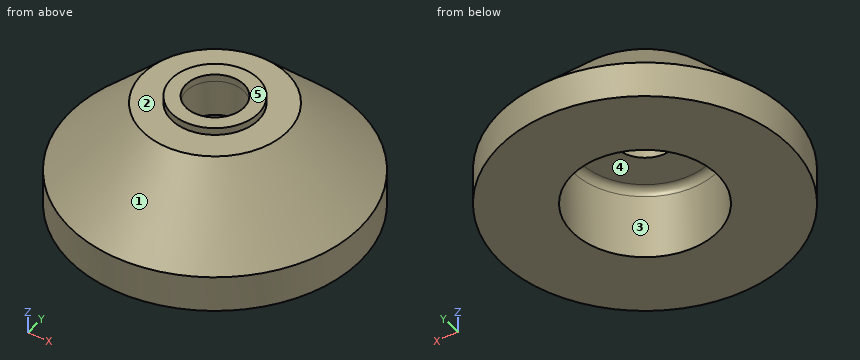
from build123d import *

# Parameters (mm, degrees)
F0_R     = 20
F1_DEPTH = 15
F2_SIZE  = 10
F3_R     = 6
F3_R_2   = 4
F4_DEPTH = 1
F5_R     = 4
F6_DEPTH = 15.001
F7_R     = 10
F8_DEPTH = 10
F9_R     = 1


with BuildPart() as f1:
    # F0 (on Top) → F1 (new body)
    with BuildSketch(Plane.XY):
        Circle(F0_R)
    extrude(amount=F1_DEPTH)

    # F2
    f2_edges = [f1.edges().sort_by_distance(p)[0] for p in [
        (-20, 0, 15),
    ]]
    chamfer(f2_edges, length=F2_SIZE)

    # F3 (on face) → F4 (join)
    with BuildSketch(Plane.XY.offset(15)):
        Circle(F3_R)
        Circle(F3_R_2, mode=Mode.SUBTRACT)
    extrude(amount=F4_DEPTH)

    # F5 (on face) → F6 (cut, through all)
    with BuildSketch(Plane.XY.offset(15)):
        Circle(F5_R)
    extrude(amount=-F6_DEPTH, mode=Mode.SUBTRACT)

    # F7 (on face) → F8 (cut)
    with BuildSketch(Plane(origin=(0, 0, 0), x_dir=(1, 0, 0), z_dir=(0, 0, -1))):
        Circle(F7_R)
    extrude(amount=-F8_DEPTH, mode=Mode.SUBTRACT)

    # F9
    f9_edges = [f1.edges().sort_by_distance(p)[0] for p in [
        (-10, 0, 10),
    ]]
    fillet(f9_edges, radius=F9_R)


solid = f1.part
The model under review builds one solid part; all positions refer to its coordinate system, in mm. Face numbers are marked on the shaded views. A direction names the side the tool comes from. Round coordinates to 2 decimals unless told otherwise and drop trailing zeros. Write each loop counter-clockwise with the first axis right and the second up, starting at its lowest first coordinate (ties: lowest second). Pieces come first, ordered by that corner, then holes. Notation, with made-up numbers: (71, 30) - (77, 30) arc R7 ccw to (77, 34) - close; hole circle Ø8 at (-10, 83.5). An arc over 180 degrees is marked (long way). One line per item, written item: value. Start each with the question number.
1. To check wall thickness, follow L1, parallel to Y at x = 0, z = 15.3; L2, parallel to Y at x = 0, z = 3; L3, parallel to Z at x = 2, y = 7. State the ranges of each line that lie inside material, in increasing order. Write a range as from..to.
2. Consider section A-A on y = 0. Write out the cut boundary in (x, z).
3. Consider section D-D on z = 12.25. Write out the cut boundary in (x, y), and give its area (3 significant figures).
4. The part is to be moulded in two halves that separate along X. For the marked faces 1, 2 and 3, say which applies: released by +X, released by -X, zero draft, split by the parting line, or undercut.
5. Clearance check with flat-ended pins moving along their axes: P1, Ø1.5, axis at x = -11.5, y = -2.5, coming from the +Z side; P2, Ø4, axis at x = -6.5, z = 13.5, coming from the +Y side; P3, Ø18, axis at x = 0, y = 0, coming from the -Z side. State where each tip first meets the part, or that it passes through.
6. Consider section C-C on z = 2. Write out the cut boundary in (x, y).
7. Machinability: for the marked faces 4 and 5, which of the approach directions +Z, -Z, +X, -X, +Y, -Y give a long, thin tool a straight path to every point of the face, cutting with its end or side? Answer none if there is none.
Checks:
1. L1: y = -6..-4, 4..6
1. L2: y = -20..-10, 10..20
1. L3: z = 10..15
2. outline: (-20, 0) - (-10, 0) - (-10, 9) arc R1 cw to (-9, 10) - (-4, 10) - (-4, 16) - (-6, 16) - (-6, 15) - (-10, 15) - (-20, 5) - close; (4, 10) - (9, 10) arc R1 cw to (10, 9) - (10, 0) - (20, 0) - (20, 5) - (10, 15) - (6, 15) - (6, 16) - (4, 16) - close
3. outline: circle Ø25.5 at (0, 0); hole circle Ø8 at (0, 0)
3. area: 460 mm^2
4. face 1: split by the parting line
4. face 2: zero draft
4. face 3: undercut
5. P1: stops at z = 13.98
5. P2: stops at y = 12.05
5. P3: stops at z = 10
6. outline: circle Ø40 at (0, 0); hole circle Ø20 at (0, 0)
7. face 4: -Z
7. face 5: +Z, +X, -X, +Y, -Y
